The drawing under review shows one solid part. Ordinate dimensions are in mm from its lowest x, y, z. Coordinates: 2 decimals unless noted, no trailing zeros. Order: outer loops, then holes, each group sorted by start corner. A loop starts at its lowest first (then second) coordinate and runs counter-clockwise, first axis right, second up.
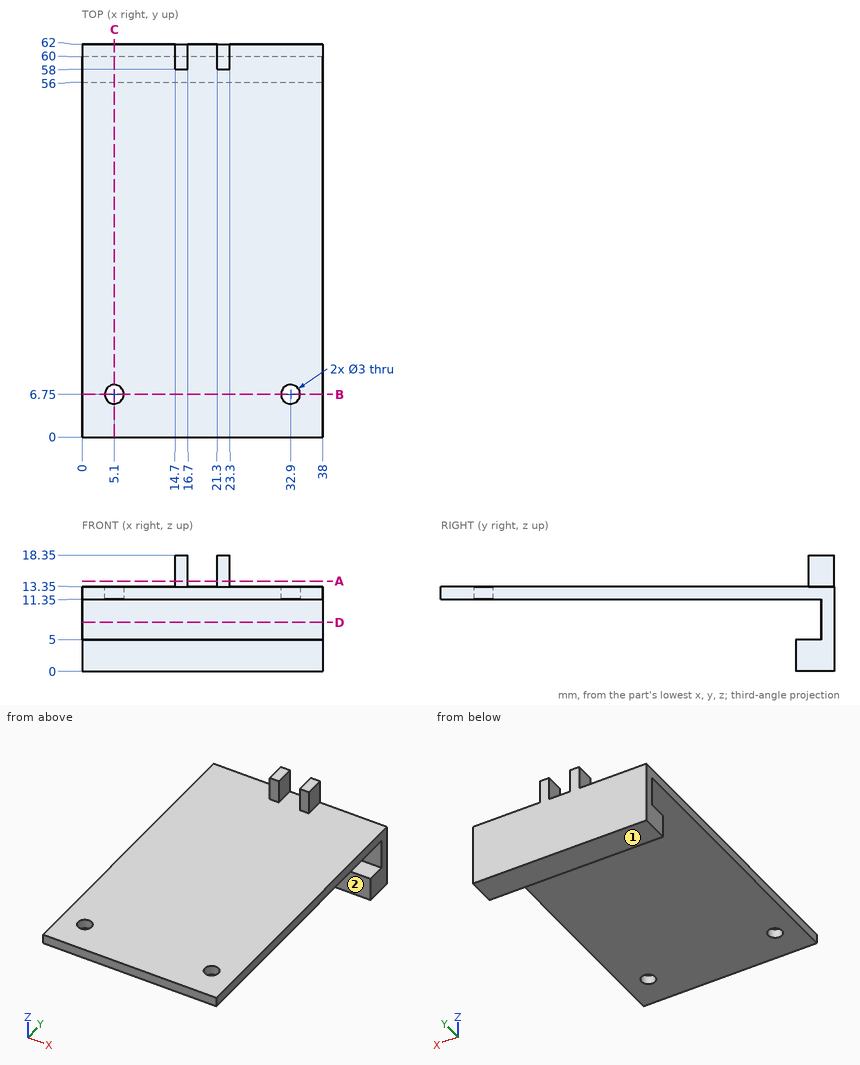
1. Add section B-B (y = 6.75). Give the boundary of the cut face in (x, z).
2. Mouldability with a two-part tool opening along Z and no side actions: class the marked faces 1 and 2 as pulls with the +Z half, pulls with the -Z half, needs draft (parallel to the pull), parting line crosses it, or undercut.
3. Insertion check: pin 1 (19 mm diameter, centred on x = 18.5, y = 15.5, fed in from -Z); pin 2 (1 mm diameter, centred on x = 22.5, z = 15.5, fed in from -Y); pin 3 (4.5 mm diameter, centred on y = 61, z = 16, fed in from +X). Each pin has a flat end and moves straight along its axis. Give the tip position at first contact, or say it passes through.
4. Add section A-A (z = 14.25). Give the boundary of the cut face in (x, y).
5. Add section D-D (z = 7.75). Give the boundary of the cut face in (x, y).
6. Add section C-C (x = 5.1). Give the boundary of the cut face in (y, z), and give its area (3 significant figures).
7. To check wall thickness, follow line 1 (Y direction, x = 5.1, z = 12.05); line 2 (Z direction, x = 30.5, y = 38); line 3 (Y direction, x = 36.5, z = 9.25). State the ranges of each line that lie inside material, in increasing order.
Solution:
1. outline: (0, 11.35) - (3.6, 11.35) - (3.6, 13.35) - (0, 13.35) - close; (6.6, 11.35) - (31.4, 11.35) - (31.4, 13.35) - (6.6, 13.35) - close; (34.4, 11.35) - (38, 11.35) - (38, 13.35) - (34.4, 13.35) - close
2. face 1: pulls with the -Z half
2. face 2: needs draft
3. pin 1: stops at z = 11.35
3. pin 2: stops at y = 58
3. pin 3: stops at x = 23.3
4. outline: (14.7, 58) - (16.7, 58) - (16.7, 62) - (14.7, 62) - close; (21.3, 58) - (23.3, 58) - (23.3, 62) - (21.3, 62) - close
5. outline: (0, 60) - (38, 60) - (38, 62) - (0, 62) - close
6. outline: (0, 11.35) - (5.25, 11.35) - (5.25, 13.35) - (0, 13.35) - close; (8.25, 11.35) - (60, 11.35) - (60, 5) - (56, 5) - (56, 0) - (62, 0) - (62, 13.35) - (8.25, 13.35) - close
6. area: 161 mm2
7. line 1: y = 0 to 5.25, 8.25 to 62
7. line 2: z = 11.35 to 13.35
7. line 3: y = 60 to 62
